Job drawing, mm, ordinate dimensions from the low corner. One solid piece. A direction names the side the tool comes from. Give positions to 0.01 mm unless a question says otherwise; leave off trailing zeros. Loops run counter-clockwise (first coordinate to the right, second up) from the corner with the lowest first, then second, coordinate; pieces in that order, holes last. Notation, with made-up numbers: M 50.25,15.25 L 66.25,15.25 A23 cw 66.25,36.25 Z; hole C 61.25,77.5 d9. An arc over 180 degrees is marked long. Put each result on its own line as item: value.
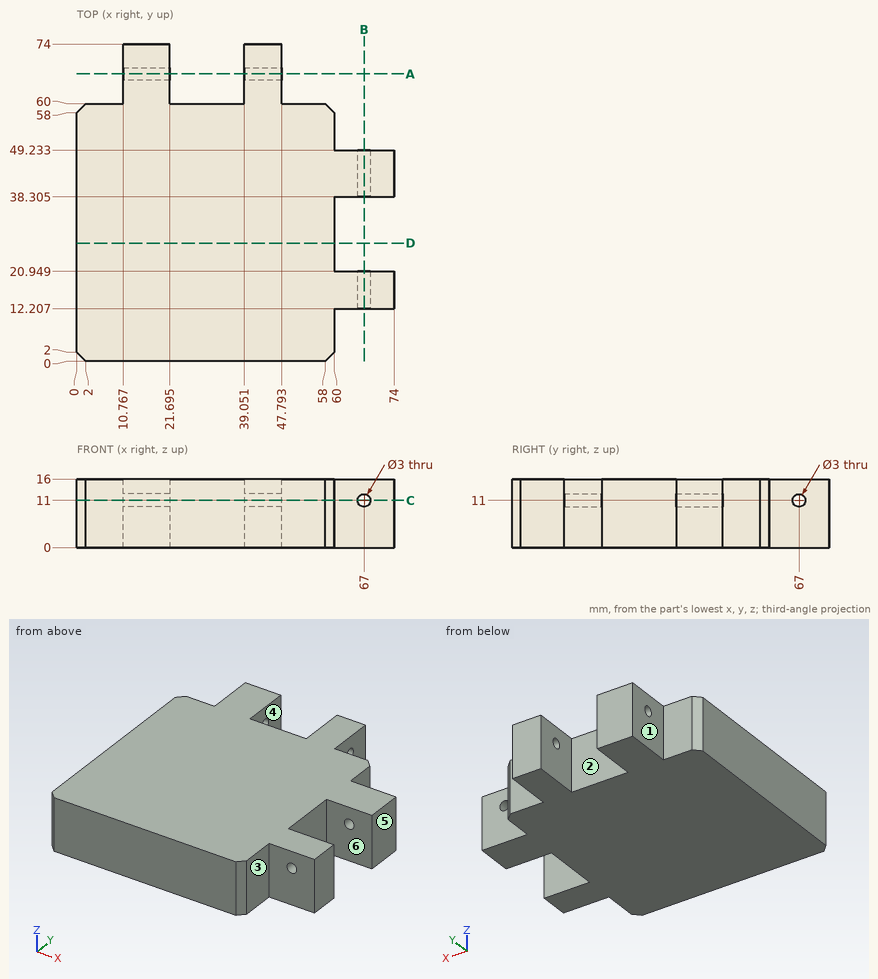
Q1. Drop flat-ended pins along their axis: pin 1 Ø4 at (y, z) = (10, 10) entering from +X; pin 2 Ø8 at (x, z) = (26, 5) entering from +Y; pin 3 Ø4 at (x, z) = (67.5, 8) entering from -Y. Give the stop position or say it passes through.
Here are the results:
pin 1: x = 60
pin 2: y = 60
pin 3: y = 12.21
Q2. Tool access for the marked faces 1, 2 and 3: list every direction of +Z, -Z, +X, -X, +Y, -Y with a clear straight run to the whole face (end or side of a thin tool).
Here are the results:
face 1: +Z, -Z, -X, +Y
face 2: +Z, -Z, +Y
face 3: +Z, -Z, +X, -Y
Q3. Slice it at B-B (x = 67). List the corners of the cut face in (y, z) (1 decimal), and give its area (3 significant figures).
Here are the results:
outline: M 12.2,0 L 20.9,0 L 20.9,9.5 L 12.2,9.5 Z; M 12.2,12.5 L 20.9,12.5 L 20.9,16 L 12.2,16 Z; M 38.3,0 L 49.2,0 L 49.2,9.5 L 38.3,9.5 Z; M 38.3,12.5 L 49.2,12.5 L 49.2,16 L 38.3,16 Z
area: 256 mm²
Q4. Slice it at C-C (z = 11). State how many separate pieces and enclosed holes the cut face has.
Here are the results:
separate pieces: 5
enclosed holes: 0
Q5. Probe line 1 (Y direction, x = 19.5, z = 11); line 2 (Z direction, x = 45, y = 67); line 3 (Y direction, x = 67, z = 7) (1 decimal). List the from-to ranges inside material, lowest first. Write a range as from..to.
Here are the results:
line 1: 0..65.5, 68.5..74
line 2: 0..9.5, 12.5..16
line 3: 12.2..20.9, 38.3..49.2
Q6. Slice it at A-A (y = 67). List the corners of the cut face in (x, z) (1 decimal), and give its area (3 significant figures).
Here are the results:
outline: M 10.8,0 L 21.7,0 L 21.7,9.5 L 10.8,9.5 Z; M 10.8,12.5 L 21.7,12.5 L 21.7,16 L 10.8,16 Z; M 39.1,0 L 47.8,0 L 47.8,9.5 L 39.1,9.5 Z; M 39.1,12.5 L 47.8,12.5 L 47.8,16 L 39.1,16 Z
area: 256 mm²
Q7. Slice it at D-D (y = 27.5). List the corners of the cut face in (x, z), and give its area (3 significant figures).
Here are the results:
outline: M 0,0 L 60,0 L 60,16 L 0,16 Z
area: 960 mm²
Q8. Mould opens along X. For the marked faces 4, 5 and 6 say: pulls with the +X half, pulls with the -X half, needs draft (parallel to the pull), parting line crosses it, or undercut.
Here are the results:
face 4: undercut
face 5: pulls with the +X half
face 6: needs draft
